Solid Edge part; units mm, degrees
sketch "Sketch1" plane through (0, 0, 0) normal (0, -1, 0) x (1, 0, 0)
  line L0 (-50, 50) -> (50, 50)
  line L1 (50, 50) -> (50, -50)
  line L2 (50, -50) -> (-50, -50)
  line L3 (-50, -50) -> (-50, 50)
  dimension "D1" = 50
  dimension "D2" = 50
extrude "Protrusion1" add sketch "Sketch1" against normal blind 25
hole "Bohrung_1" at (0, 0, 0) direction (0, 1, 0) diameter 30 end up to next
hole "Bohrung_2" at (-30, 0, 30) direction (0, 1, 0) diameter 6 end up to next
hole "Hole1" at (30, 0, 30) direction (0, 1, 0) diameter 6 end up to next
hole "Hole2" at (30, 0, -30) direction (0, 1, 0) diameter 6 end up to next
hole "Hole3" at (-30, 0, -30) direction (0, 1, 0) diameter 6 end up to next
hole "Bohrung_6" at (25, 25, 0) direction (0, -1, 0) diameter 6.6 end up to next countersink diameter 13.71 countersink angle 90
hole "Hole4" at (-12.5, 25, 21.6506) direction (0, -1, 0) diameter 6.6 end up to next countersink diameter 13.71 countersink angle 90
hole "Hole5" at (-12.5, 25, -21.6506) direction (0, -1, 0) diameter 6.6 end up to next countersink diameter 13.71 countersink angle 90
sketch "Sketch2" plane through (0, 25, 0) normal (0, 1, 0) x (-1, 0, 0)
  circle A0 centre (-30, 30) radius 6
  circle A1 centre (30, 30) radius 6
  circle A2 centre (30, -30) radius 6
  circle A3 centre (-30, -30) radius 6
extrude "Extrusionsausschnitt_2" cut sketch "Sketch2" against normal blind 5
sketch "Sketch3" plane through (0, 25, 0) normal (0, 1, 0) x (-1, 0, 0)
  line L0 (-25, 50) -> (-10, 35)
  line L1 (-10, 35) -> (10, 35)
  line L2 (10, 35) -> (25, 50)
  line L3 (25, 50) -> (-25, 50)
  line L4 (50, 25) -> (35, 10)
  line L5 (35, 10) -> (35, -10)
  line L6 (35, -10) -> (50, -25)
  line L7 (50, 25) -> (50, -25)
  line L8 (25, -50) -> (10, -35)
  line L9 (10, -35) -> (-10, -35)
  line L10 (-10, -35) -> (-25, -50)
  line L11 (-25, -50) -> (25, -50)
extrude "Extrusionsausschnitt_3" cut sketch "Sketch3" against normal blind 2384.1506
fillet "Verrundung_1" radius 20 4 edges at (50, 12.5, 50) (-50, 12.5, 50) (-50, 12.5, -50) (50, 12.5, -50)
fillet "Verrundung_2" radius 10 12 edges at (-10, 12.5, 35) (10, 12.5, 35) (-25, 12.5, 50) (25, 12.5, 50) (-50, 12.5, 25) (-35, 12.5, 10) (-35, 12.5, -10) (-50, 12.5, -25) (-25, 12.5, -50) (-10, 12.5, -35) (10, 12.5, -35) (25, 12.5, -50)
CAD build for the part. Positions are in the model's coordinates, mm. A direction names the side the tool comes from. Give positions to 0.01 mm unless a question says otherwise; leave off trailing zeros. Loops run counter-clockwise (first coordinate to the right, second up) from the corner with the lowest first, then second, coordinate; pieces in that order, holes last. Notation, with made-up numbers: M 58,24.25 L 85,24.25 A19 ccw 85,43.25 Z; hole C 7,70.25 d11. An arc over 180 degrees is marked long. Write each question's results on one line, items separated by ' | '.
Q1. Band-saw the part on B-B on y = 11.5. Give the number of separate pieces and of enclosed holes in the cut face, and give its area (3 significant figures).
Geometry check:
separate pieces: 1 | enclosed holes: 8 | area: 7,160 mm²
Q2. Which spindle directions (+Z, -Z, +X, -X, +Y, -Y) get a long thin tool onto all of the face, cutting with end or side? Do faces 4 (the face through (-25.24, 22.54, -33.65)), 5 (the face through (-42, 13, -17)), 6 (the face through (18, 13, 43)). Say none if no direction does.
Geometry check:
face 4: +Y | face 5: -X, +Y, -Y | face 6: +Z, +Y, -Y
Q3. Probe probe 1 along Z at (x, y) = (-30, 21.15); probe 2 along X at (y, z) = (3.75, 30.5); probe 3 along Z at (x, y) = (-31.5, 6.25). List the from-to ranges inside material, lowest first.
Geometry check:
probe 1: z = -50 to -36, -24 to 24, 36 to 50 | probe 2: x = -49.99 to -32.96, -27.04 to 27.04, 32.96 to 49.99 | probe 3: z = -49.94 to -32.6, -27.4 to 27.4, 32.6 to 49.94
Q4. Band-saw the part on C-C on x = 40.5. Write the cut outline in (y, z).
Geometry check:
outline: M 0,-47.02 L 25,-47.02 L 25,47.02 L 0,47.02 Z
Q5. Flat gauge pins, fed straight in: P1, Ø5, axis at x = 30, z = 30, coming from the +Y side; P2, Ø6, axis at x = -32.5, z = -30.5, coming from the +Y side; P3, Ø13, axis at x = 0.5, y = 10, coming from the -Z side; P4, Ø10, axis at x = -16, y = 14, coming from the +Z side. Where does each tip first touch, or does it go through?
Geometry check:
P1: passes through | P2: stops at y = 20 | P3: stops at z = -35.07 | P4: stops at z = 46
Q6. Band-saw the part on A-A on z = 0. Write the cut outline in (x, y) (3 decimals).
Geometry check:
outline: M -35,0 L -15,0 L -15,25 L -35,25 Z; M 15,0 L 21.7,0 L 21.7,21.445 L 18.145,25 L 15,25 Z; M 28.3,0 L 50,0 L 50,25 L 31.855,25 L 28.3,21.445 Z
Q7. Mould opens along X. For faces 1 (the face through (-44.297, 12.675, 43.986)), 2 (the face through (44.297, 12.675, -43.986)), 3 (the face through (17, 13, -42)) say: pulls with the +X half, pulls with the -X half, needs draft (parallel to the pull), parting line crosses it, or undercut.
Geometry check:
face 1: pulls with the -X half | face 2: pulls with the +X half | face 3: undercut
